Build history of the part. All positions in model axes, mm. A direction names the side the tool comes from. Give positions to 0.01 mm unless a question says otherwise; leave off trailing zeros. Order: outer loops, then holes, each group sorted by start corner. A loop starts at its lowest first (then second) coordinate and runs counter-clockwise, first axis right, second up. Notation, with made-up numbers: (73, -6.75) - (125, -6.75) arc R32 ccw to (125, 23.25) - close; hole circle Ø6 at (-0.5, 88). An arc over 180 degrees is marked (long way). One line per item, written item: value.
Autodesk Inventor part; units mm, degrees
ref_plane "YZ Plane" through (0, 0, 0) normal (1, 0, 0) x (0, 1, 0)
ref_plane "XZ Plane" through (0, 0, 0) normal (0, 1, 0) x (-1, 0, 0)
ref_plane "XY Plane" through (0, 0, 0) normal (0, 0, 1) x (1, 0, 0)
sketch "Sketch1" plane through (0, 0, 0) normal (0, 0, 1) x (1, 0, 0)
  line L0 (0, 0) -> (7.112, 0)
  line L1 (7.112, 0) -> (7.112, 4.5212)
  line L2 (7.112, 4.5212) -> (0, 4.5212)
  line L3 (0, 4.5212) -> (0, 0)
  dimension "d0" = 7.112
  dimension "d1" = 4.5212
extrude "Extrusion1" add sketch "Sketch1" along normal blind 10.16
sketch "Sketch2" plane through (0, 0, 10.16) normal (0, 0, 1) x (1, 0, 0)
  line L0 (0.6954, 3.8901) -> (6.5198, 3.8901)
  line L1 (6.5198, 3.8901) -> (6.5198, 0.5433)
  line L2 (6.5198, 0.5433) -> (0.6954, 0.5433)
  line L3 (0.6954, 0.5433) -> (0.6954, 3.8901)
  point P0 (0, 0)
extrude "Extrusion2" cut sketch "Sketch2" against normal blind 10.16
properties part number "connection"
(1) Slice it at A-A, the plane y = 2.95. Give the cut face in (x, z).
Completed:
outline: (0, 0) - (0.7, 0) - (0.7, 10.16) - (0, 10.16) - close; (6.52, 0) - (7.11, 0) - (7.11, 10.16) - (6.52, 10.16) - close
(2) Pull direction Y, two halves, no side cores. Call faces 1 (the face through (4, 0.543, 5)), 2 (the face through (4, 4.521, 5)), 3 (the face through (3.5, 4.3, 0)): +Y half, -Y half, draft (parallel to the pull), parting line (faces both ways), or undercut.
Completed:
face 1: undercut
face 2: +Y half
face 3: draft
(3) 3-axis set-ups, long thin cutter, end or side, ignore diameter. For faces 4 (the face through (4, 3.89, 5)), 5 (the face through (4, 0, 5)): which of +Z, -Z, +X, -X, +Y, -Y reach the whole face in a straight line?
Completed:
face 4: +Z, -Z
face 5: +Z, -Z, +X, -X, -Y
(4) Slice it at B-B, the plane x = 5.25. Give the cut face in (y, z).
Completed:
outline: (0, 0) - (0.54, 0) - (0.54, 10.16) - (0, 10.16) - close; (3.89, 0) - (4.52, 0) - (4.52, 10.16) - (3.89, 10.16) - close
(5) Pin check, flat tip, straight feed: P1, Ø1.5, axis at x = 5.5, y = 3, coming from the +Z side. Stop position of the tip, or through.
Completed:
P1: through
(6) Drill centre lines: line 1 (Y direction, x = 5, z = 3.25); line 2 (X direction, y = 2.55, z = 0.5). Where is each one in solid material? Low to high.
Completed:
line 1: 0 to 0.54, 3.89 to 4.52
line 2: 0 to 0.7, 6.52 to 7.11
(7) Slice it at C-C, the plane z = 1. Give the cut face in (x, y).
Completed:
outline: (0, 0) - (7.11, 0) - (7.11, 4.52) - (0, 4.52) - close; hole (0.7, 0.54) - (6.52, 0.54) - (6.52, 3.89) - (0.7, 3.89) - close
